Could you check a few things on this model? Use its own coordinates, in mm. Coordinates: 2 decimals unless noted, no trailing zeros. Order: outer loops, then holes, each group sorted by start corner. A loop starts at its lowest first (then second) coordinate and runs counter-clockwise, first axis right, second up. Notation, with made-up numbers: (88.5, 32.5) -> (100.5, 32.5) arc R11 ccw to (100.5, 53.5) -> close; hole circle Ø6 at (16, 74.5). An arc over 180 degrees is marked (long way). Put each result on its own line as item: value. Start each with the question number.
Q1. If we section it at B-B (y = 8.5): Please give me the cut outline in (x, z).
Q2. If we section it at D-D (z = 4): Please give me the cut outline in (x, y).
Q3. Please list where these lines run through material, in increasing order: line 1 along X through (y, z) = (-10, 35.5); line 2 along Z through (x, y) = (-7.5, 13.5); line 3 along X through (y, z) = (8.5, 32.5).
Q4. If we section it at A-A (x = 0): Please give me the cut outline in (y, z), and give its area (3 significant figures).
Q5. If we section it at C-C (x = -6): Please give me the cut outline in (y, z).
Q6. Will these pins go through, and if not, where does the flat tip stop? pin 1 (12 mm diameter, centred on y = -15, z = 32, fed in from -X); pin 2 (7 mm diameter, centred on x = 11.99, y = -0.36, fed in from +Z); pin 3 (6 mm diameter, centred on y = -7.5, z = 12.5, fed in from -X); pin 4 (8 mm diameter, centred on y = -0.5, z = 12, fed in from +X).
Q7. We'd pull the mould along Y, two halves only. Please class faces 1 (the face through (-14.766, 1.506, 35.07)), 2 (the face through (-4, -4, 30)), 3 (the face through (-1.08, -4.88, 15.21)): +Y half, -Y half, draft (parallel to the pull), parting line (faces both ways), or undercut.
from build123d import *

# Parameters (mm, degrees)
SKETCH001_R        = 3
POCKET_DEPTH       = 10
POLARPATTERN_COUNT = 6


with BuildPart() as part:
    # Sketch → Revolution (revolve)
    with BuildSketch(Plane.XZ):
        Polygon((0, 0), (5, 0), (5, 30), (20, 30), (20, 40), (0, 40), align=None)
    revolve(axis=Axis((0, 0, 0), (0, 0, 1)))

    # Sketch001 (on Face5 of Revolution) → Pocket (cut)
    with BuildSketch(Plane.XY.offset(40)):
        with Locations((-5.688479, 10.56604)):
            Circle(SKETCH001_R)
    pocket = extrude(amount=-POCKET_DEPTH, mode=Mode.SUBTRACT)

    # PolarPattern: Pocket ×6 about axis
    polarpattern_axis = Axis((0, 0, 40), (0, 0, 1))
    for i in range(1, POLARPATTERN_COUNT):
        add(pocket.rotate(polarpattern_axis, i * 360 / POLARPATTERN_COUNT), mode=Mode.SUBTRACT)


solid = part.part
The answers:
1. outline: (-18.1, 30) -> (-7.86, 30) -> (-7.86, 40) -> (-18.1, 40) -> close; (-3.51, 30) -> (3.84, 30) -> (3.84, 40) -> (-3.51, 40) -> close; (8.77, 30) -> (18.1, 30) -> (18.1, 40) -> (8.77, 40) -> close
2. outline: circle Ø10 at (0, 0)
3. line 1: -17.32 to -9.3, -3.31 to 2.74, 8.63 to 17.32
3. line 2: 30 to 40
3. line 3: -18.1 to -7.86, -3.51 to 3.84, 8.77 to 18.1
4. outline: (-20, 30) -> (-5, 30) -> (-5, 0) -> (5, 0) -> (5, 30) -> (20, 30) -> (20, 40) -> (-20, 40) -> close
4. area: 700 mm^2
5. outline: (-19.08, 30) -> (-13.19, 30) -> (-13.19, 40) -> (-19.08, 40) -> close; (-7.23, 30) -> (7.58, 30) -> (7.58, 40) -> (-7.23, 40) -> close; (13.55, 30) -> (19.08, 30) -> (19.08, 40) -> (13.55, 40) -> close
6. pin 1: x = -17.86
6. pin 2: z = 40
6. pin 3: x = -2.18
6. pin 4: x = 5
7. face 1: undercut
7. face 2: draft
7. face 3: parting line
